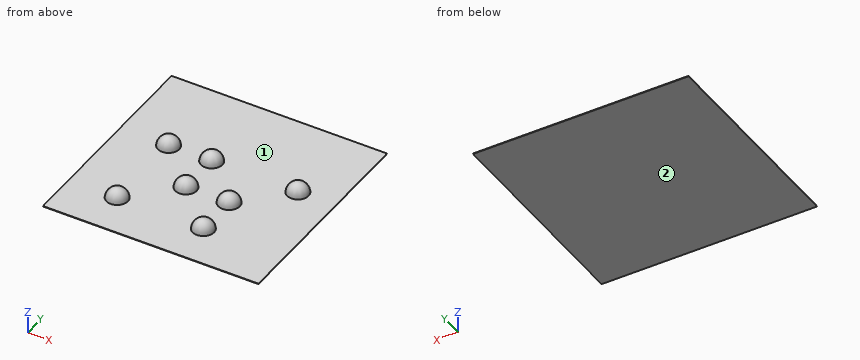
```python
from build123d import *

# Parameters (mm, degrees)
F1_W     = 200
F1_H     = 200
F1_R     = 10
F2_DEPTH = 0.5
F3_DEPTH = 10


# Not quite as in the source:
# - a fillet or chamfer that OpenCascade refuses, or shapes differently, is made with other operations: its cross-section is extruded or revolved along the edge and cut away or added


with BuildPart() as f2:
    # F1 (on face) → F2 (new body)
    with BuildSketch(Plane.XY):
        Rectangle(F1_W, F1_H)
        with Locations((-55, -60)):
            Circle(F1_R, mode=Mode.SUBTRACT)
        with Locations((-15, -20)):
            Circle(F1_R, mode=Mode.SUBTRACT)
        with Locations((25, -60)):
            Circle(F1_R, mode=Mode.SUBTRACT)
        with Locations((25, -20)):
            Circle(F1_R, mode=Mode.SUBTRACT)
        with Locations((-55, 20)):
            Circle(F1_R, mode=Mode.SUBTRACT)
        with Locations((-15, 20)):
            Circle(F1_R, mode=Mode.SUBTRACT)
        with Locations((65, 20)):
            Circle(F1_R, mode=Mode.SUBTRACT)
    extrude(amount=F2_DEPTH)

    # F1 (on face) → F3 (join)
    with BuildSketch(Plane.XY):
        with Locations((-55, -60)):
            Circle(F1_R)
        with Locations((-55, 20)):
            Circle(F1_R)
        with Locations((-15, -20)):
            Circle(F1_R)
        with Locations((-15, 20)):
            Circle(F1_R)
        with Locations((25, -60)):
            Circle(F1_R)
        with Locations((25, -20)):
            Circle(F1_R)
        with Locations((65, 20)):
            Circle(F1_R)
    extrude(amount=F3_DEPTH)

    # F4: fillet of radius 10 on 7 edges, made by hand

    # F4_s1 → F4_t2 (revolve, cut)
    with BuildSketch(Plane.XZ.offset(-20)):
        with BuildLine():
            ThreePointArc((-45, 0.5), (-48.0954678017, 7.2456883731), (-54.9874921777, 10))
            Line((-54.9874921777, 10), (-45, 10))
            Line((-45, 10), (-45, 0.5))
        make_face()
    revolve(axis=Axis((-55, 20, 10), (0, 0, 1)), mode=Mode.SUBTRACT)

    # F4_s3 → F4_t4 (revolve, cut)
    with BuildSketch(Plane.XZ.offset(-20)):
        with BuildLine():
            ThreePointArc((-5, 0.5), (-8.0954678017, 7.2456883731), (-14.9874921777, 10))
            Line((-14.9874921777, 10), (-5, 10))
            Line((-5, 10), (-5, 0.5))
        make_face()
    revolve(axis=Axis((-15, 20, 10), (0, 0, 1)), mode=Mode.SUBTRACT)

    # F4_s5 → F4_t6 (revolve, cut)
    with BuildSketch(Plane.XZ.offset(-20)):
        with BuildLine():
            ThreePointArc((75, 0.5), (71.9045321983, 7.2456883731), (65.0125078223, 10))
            Line((65.0125078223, 10), (75, 10))
            Line((75, 10), (75, 0.5))
        make_face()
    revolve(axis=Axis((65, 20, 10), (0, 0, 1)), mode=Mode.SUBTRACT)

    # F4_s7 → F4_t8 (revolve, cut)
    with BuildSketch(Plane.XZ.offset(20)):
        with BuildLine():
            ThreePointArc((35, 0.5), (31.9045321983, 7.2456883731), (25.0125078223, 10))
            Line((25.0125078223, 10), (35, 10))
            Line((35, 10), (35, 0.5))
        make_face()
    revolve(axis=Axis((25, -20, 10), (0, 0, 1)), mode=Mode.SUBTRACT)

    # F4_s9 → F4_t10 (revolve, cut)
    with BuildSketch(Plane.XZ.offset(20)):
        with BuildLine():
            ThreePointArc((-5, 0.5), (-8.0954678017, 7.2456883731), (-14.9874921777, 10))
            Line((-14.9874921777, 10), (-5, 10))
            Line((-5, 10), (-5, 0.5))
        make_face()
    revolve(axis=Axis((-15, -20, 10), (0, 0, 1)), mode=Mode.SUBTRACT)

    # F4_s11 → F4_t12 (revolve, cut)
    with BuildSketch(Plane.XZ.offset(60)):
        with BuildLine():
            ThreePointArc((-45, 0.5), (-48.0954678017, 7.2456883731), (-54.9874921777, 10))
            Line((-54.9874921777, 10), (-45, 10))
            Line((-45, 10), (-45, 0.5))
        make_face()
    revolve(axis=Axis((-55, -60, 10), (0, 0, 1)), mode=Mode.SUBTRACT)

    # F4_s13 → F4_t14 (revolve, cut)
    with BuildSketch(Plane.XZ.offset(60)):
        with BuildLine():
            ThreePointArc((35, 0.5), (31.9045321983, 7.2456883731), (25.0125078223, 10))
            Line((25.0125078223, 10), (35, 10))
            Line((35, 10), (35, 0.5))
        make_face()
    revolve(axis=Axis((25, -60, 10), (0, 0, 1)), mode=Mode.SUBTRACT)


solid = f2.part
```
Geometry: final body of the model. Coordinates: model frame, mm. Face numbers are marked on the shaded views. A direction names the side the tool comes from. Round coordinates to 2 decimals unless told otherwise and drop trailing zeros. Write each loop counter-clockwise with the first axis right and the second up, starting at its lowest first coordinate (ties: lowest second). Pieces come first, ordered by that corner, then holes. Notation, with made-up numbers: (-32, 10) -> (-6, 10) arc R21 ccw to (-6, 15) -> close; hole circle Ø1 at (-30, 13.25). An arc over 180 degrees is marked (long way). Use CSV: the item, a comma, the result in double quotes. Start each with the question number.
Q1. Section A-A (z = 7.25). Give the number of separate pieces and of enclosed holes in the cut face, plus the area to 3 significant figures.
Q2. First-contact query: pin 1 Ø2 at (x, z) = (-42, 2) entering from +Y; pin 2 Ø2 at (x, z) = (25, 7) entering from +Y. Flat tips, straight axial feed; report the tip coordinate or a pass-through.
Q3. Line query: L1, parallel to Z at x = 39.5, y = -47.5; L2, parallel to Y at x = 20.5, z = 4.25; L3, parallel to X at y = 14.5, z = 6.5. Output: solid intervals per line, ascending.
Q4. Section B-B (x = -69). Return loops of the section in (y, z), plus the area to 3 significant figures.
Q5. Reachability of the marked faces 1 and 2 from +Z, -Z, +X, -X, +Y, -Y: full face, straight path, thin tool, end or side. Return the list, or none.
Result sheet:
1,separate pieces,"7"
1,enclosed holes,"0"
1,area,"1,050 mm²"
2,pin 1,"through"
2,pin 2,"y = -11.99"
3,L1,"0 to 0.5"
3,L2,"-67.87 to -52.13, -27.87 to -12.13"
3,L3,"-60.26 to -49.74, -20.26 to -9.74, 59.74 to 70.26"
4,outline,"(-100, 0) -> (100, 0) -> (100, 0.5) -> (-100, 0.5) -> close"
4,area,"100 mm²"
5,face 1,"+Z"
5,face 2,"-Z, +X, -X, +Y, -Y"
